Could you check a few things on this model? Use its own coordinates, in mm. Give positions to 0.01 mm unless a question says otherwise; leave off trailing zeros. Loops run counter-clockwise (first coordinate to the right, second up) from the corner with the lowest first, then second, coordinate; pieces in that order, holes last. Notation, with made-up numbers: (39.5, 52) -> (77.5, 52) arc R29 ccw to (77.5, 89) -> close; hole circle Ø9 at (41, 26). An arc over 180 degrees is marked (long way). Put each result on its own line as item: value.
Autodesk Inventor part; units mm, degrees
ref_plane "YZ Plane" through (0, 0, 0) normal (1, 0, 0) x (0, 1, 0)
ref_plane "XZ Plane" through (0, 0, 0) normal (0, 1, 0) x (-1, 0, 0)
ref_plane "XY Plane" through (0, 0, 0) normal (0, 0, 1) x (1, 0, 0)
sketch "Sketch1" plane through (0, 0, 0) normal (0, 0, 1) x (1, 0, 0)
  circle A0 centre (0, 0) radius 15
  line L0 (0, 0) -> (-49, 0) construction
  circle A1 centre (-49, 0) radius 10
  line L1 (-50.0204, 9.9478) -> (-1.5306, 14.9217)
  line L2 (-50.0204, -9.9478) -> (-1.5306, -14.9217)
  dimension "d0" = 20
  dimension "d1" = 30
  dimension "d2" = 49
extrude "Extrusion1" add sketch "Sketch1" along normal mid plane 3.5
sketch "Sketch2" plane through (0, 0, 1.75) normal (0, 0, 1) x (1, 0, 0)
  arc A0 (-1.5306, -14.9217) -> (-1.5306, 14.9217) centre (0, 0) ccw
hole "Hole1" at (0, 0, 1.75) direction (0, 0, -1) diameter 15.84 end through all
sketch "Sketch3" plane through (0, 0, 1.75) normal (0, 0, 1) x (1, 0, 0)
  arc A0 (-50.0204, 9.9478) -> (-50.0204, -9.9478) centre (-49, 0) ccw
hole "Hole2" at (-49, 0, 1.75) direction (0, 0, -1) diameter 9 end through all
properties part number "313-01-02" material "Steel"
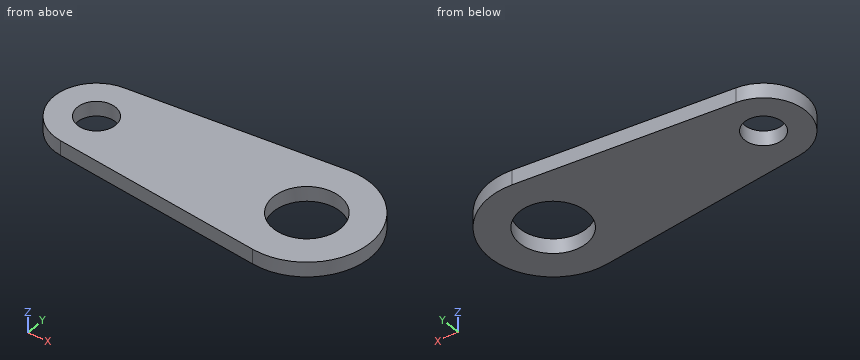
1. If we section it at C-C (z = -0.8): List the corners of the cut face in (x, y) for me.
Recorded:
outline: (-50.02, -9.95) -> (-1.53, -14.92) arc R15 ccw (long way) to (-1.53, 14.92) -> (-50.02, 9.95) arc R10 ccw to start; hole circle Ø9 at (-49, 0); hole circle Ø15.84 at (0, 0)
2. If we section it at B-B (x = 0): List the corners of the cut face in (y, z) for me.
Recorded:
outline: (-15, -1.75) -> (-7.92, -1.75) -> (-7.92, 1.75) -> (-15, 1.75) -> close; (7.92, -1.75) -> (15, -1.75) -> (15, 1.75) -> (7.92, 1.75) -> close
3. If we section it at D-D (y = -7): List the corners of the cut face in (x, z) for me.
Recorded:
outline: (-56.14, -1.75) -> (-3.7, -1.75) -> (-3.7, 1.75) -> (-56.14, 1.75) -> close; (3.7, -1.75) -> (13.27, -1.75) -> (13.27, 1.75) -> (3.7, 1.75) -> close
4. If we section it at A-A (y = 0): List the corners of the cut face in (x, z) for me, then the cut area to 3 significant figures.
Recorded:
outline: (-59, -1.75) -> (-53.5, -1.75) -> (-53.5, 1.75) -> (-59, 1.75) -> close; (-44.5, -1.75) -> (-7.92, -1.75) -> (-7.92, 1.75) -> (-44.5, 1.75) -> close; (7.92, -1.75) -> (15, -1.75) -> (15, 1.75) -> (7.92, 1.75) -> close
area: 172 mm^2
5. I need wall thicknesses on line 1 (Y direction, x = 0, z = 0.3); line 2 (X direction, y = -3, z = 1.35); line 3 (X direction, y = 2.5, z = -1.3). Which ranges of each line are inside material? Lowest first, please.
Recorded:
line 1: y = -15 to -7.92, 7.92 to 15
line 2: x = -58.54 to -52.35, -45.65 to -7.33, 7.33 to 14.7
line 3: x = -58.68 to -52.74, -45.26 to -7.52, 7.52 to 14.79
